from build123d import *

# Parameters (mm, degrees)
BOSS_EXTRUDE1_DEPTH = 15
SKETCH4_W           = 5
SKETCH4_H           = 40
BOSS_EXTRUDE2_DEPTH = 1.5
SKETCH5_W           = 5
SKETCH5_H           = 40
BOSS_EXTRUDE3_DEPTH = 1.5
SKETCH6_W           = 8
SKETCH6_H           = 15
BOSS_EXTRUDE4_DEPTH = 45
SKETCH7_W           = 5
SKETCH7_H           = 10
BOSS_EXTRUDE5_DEPTH = 5
SKETCH8_W           = 5
SKETCH8_H           = 10
BOSS_EXTRUDE6_DEPTH = 5


with BuildPart() as part:
    # Sketch2 → Boss-Extrude1 (new body)
    with BuildSketch(Plane(origin=(0, 0, 0), x_dir=(1, 0, 0), z_dir=(0, 1, 0))):
        with BuildLine():
            Line((0, 0), (0, 40))
            Line((0, 40), (5, 40))
            Line((5, 40), (5, 37))
            Line((5, 37), (55, 37))
            Line((55, 37), (55, 39.5))
            Line((55, 39.5), (56.5, 39.5))
            ThreePointArc((56.5, 39.5), (62.264260255, 37.258522387), (65, 31.711753397))
            Line((65, 31.711753397), (65, 26.711753397))
            Line((65, 26.711753397), (15, 19.51828483))
            Line((15, 19.51828483), (15, 3))
            Line((15, 3), (5, 3))
            Line((5, 3), (5, 0))
            Line((5, 0), (0, 0))
        make_face()
    extrude(amount=BOSS_EXTRUDE1_DEPTH)

    # Sketch4 → Boss-Extrude2 (add)
    with BuildSketch(Plane(origin=(0, 15, 0), x_dir=(1, 0, 0), z_dir=(0, 1, 0))):
        with Locations((2.5, 20)):
            Rectangle(SKETCH4_W, SKETCH4_H)
    extrude(amount=BOSS_EXTRUDE2_DEPTH)

    # Sketch5 → Boss-Extrude3 (add)
    with BuildSketch(Plane.XZ):
        with Locations((2.5, -20)):
            Rectangle(SKETCH5_W, SKETCH5_H)
    extrude(amount=BOSS_EXTRUDE3_DEPTH)

    # Sketch6 → Boss-Extrude4 (add)
    with BuildSketch(Plane(origin=(15, 0, 0), x_dir=(0, 0, -1), z_dir=(1, 0, 0))):
        with Locations((7, 7.5)):
            Rectangle(SKETCH6_W, SKETCH6_H)
    extrude(amount=BOSS_EXTRUDE4_DEPTH)

    # Sketch7 → Boss-Extrude5 (add)
    with BuildSketch(Plane.XY):
        with Locations((2.5, 7.5)):
            Rectangle(SKETCH7_W, SKETCH7_H)
    extrude(amount=BOSS_EXTRUDE5_DEPTH)

    # Sketch8 → Boss-Extrude6 (add)
    with BuildSketch(Plane(origin=(0, 0, -40), x_dir=(-1, 0, 0), z_dir=(0, 0, -1))):
        with Locations((-2.5, 7.5)):
            Rectangle(SKETCH8_W, SKETCH8_H)
    extrude(amount=BOSS_EXTRUDE6_DEPTH)


solid = part.part
Work out the finished part from the listing and answer in its coordinate system (mm). A direction names the side the tool comes from. Give positions to 0.01 mm unless a question says otherwise; leave off trailing zeros. Loops run counter-clockwise (first coordinate to the right, second up) from the corner with the lowest first, then second, coordinate; pieces in that order, holes last. Notation, with made-up numbers: (-14, 67.25) -> (43, 67.25) arc R7 ccw to (43, 71.25) -> close; hole circle Ø10 at (13, 60). An arc over 180 degrees is marked (long way). Use a Markdown table: item, result. Add a question column.
1) The part is cut by section A-A, the plane y = 13.25. Determine the outline of the cut face in (x, z), plus the area to 3 significant figures.
2) The part is cut by section C-C, the plane z = -5. Determine the outline of the cut face in (x, y).
3) The part is cut by section B-B, the plane x = 20. Determine the outline of the cut face in (y, z), plus the area to 3 significant figures.
4) Which of the six approach directions +Z, -Z, +X, -X, +Y, -Y give full straight-line access (tool end or side, diameter ignored) to faces 1 (the flat face through (5, 16, -26)), 2 (the flat face through (55, 7, -38)), 3 (the flat face through (3, 12.5, -42)), 4 (the flat face through (3, 2.5, -42)), 5 (the flat face through (28, 15, -25))?
5) For a pull along Z with two mould halves and no side action, classify faces 6 (the flat face through (2, 1, -40)), 7 (the flat face through (2, -1.5, -20)), 8 (the flat face through (40.35, 7.395, -23.165)), 9 (the flat face through (37, 7, -11)) as +Z half, -Z half, draft (parallel to the pull), parting line (faces both ways), or undercut.
6) Consider line 1 along X through (y, z) = (10.5, -1); line 2 along Y through (x, z) = (13, -19). Determine where each line is inside the solid, lowest interval first.
7) Each of these flat-tipped pins is pushed along its axis until it touches: P1, Ø1.5, axis at x = 34, y = 13.5, coming from the -Z side; P2, Ø12, axis at x = 17, z = -23.5, coming from the +Y side; P3, Ø2, axis at x = 2, y = 0.5, coming from the +Z side. Where does it stop, or does it pass through?
8) The part is cut by section D-D, the plane x = 27.5. Determine the outline of the cut face in (y, z).
Reported:
| question | item | result |
|---|---|---|
| 1 | outline | (0, -40) -> (5, -40) -> (5, -37) -> (55, -37) -> (55, -39.5) -> (56.5, -39.5) arc R8.53 ccw to (65, -31.71) -> (65, -26.71) -> (15, -19.52) -> (15, -11) -> (60, -11) -> (60, -3) -> (5, -3) -> (5, 0) -> (0, 0) -> close |
| 1 | area | 1,600 mm^2 |
| 2 | outline | (0, -1.5) -> (5, -1.5) -> (5, 0) -> (60, 0) -> (60, 15) -> (5, 15) -> (5, 16.5) -> (0, 16.5) -> close |
| 3 | outline | (0, -37) -> (15, -37) -> (15, -20.24) -> (0, -20.24) -> close; (0, -11) -> (15, -11) -> (15, -3) -> (0, -3) -> close |
| 3 | area | 371 mm^2 |
| 4 | face 1 | none |
| 4 | face 2 | -Z, +Y, -Y |
| 4 | face 3 | -Z, +X, -X, +Y |
| 4 | face 4 | -Z, +X, -X, -Y |
| 4 | face 5 | +Z, -Z, +X, +Y |
| 5 | face 6 | -Z half |
| 5 | face 7 | draft |
| 5 | face 8 | undercut |
| 5 | face 9 | undercut |
| 6 | line 1 | x = 0 to 5 |
| 6 | line 2 | y = 0 to 15 |
| 7 | P1 | stops at z = -37 |
| 7 | P2 | stops at y = 15 |
| 7 | P3 | stops at z = 0 |
| 8 | outline | (0, -37) -> (15, -37) -> (15, -21.32) -> (0, -21.32) -> close; (0, -11) -> (15, -11) -> (15, -3) -> (0, -3) -> close |
